Here's how the part is built. I have some questions about the finished solid (model axes, mm). Face numbers are marked on the shaded views. A direction names the side the tool comes from. Round coordinates to 2 decimals unless told otherwise and drop trailing zeros. Order: outer loops, then holes, each group sorted by start corner. A loop starts at its lowest first (then second) coordinate and runs counter-clockwise, first axis right, second up.
```python
from build123d import *

# Parameters (mm, degrees)
ESQUISSE1_R             = 40
ESQUISSE1_R_2           = 10
BOSS_EXTRU_1_DEPTH      = 12.5
ESQUISSE2_R             = 22.5
ENL_V_MAT_EXTRU_1_DEPTH = 5
CHANFREIN1_SIZE         = 5
ESQUISSE4_R             = 3
ENL_V_MAT_EXTRU_2_DEPTH = 61
BOSS_EXTRU_2_DEPTH      = 2
BOSS_EXTRU_2_DEPTH_BACK = 17
ESQUISSE5_R             = 11
ESQUISSE5_R_2           = 10
CHANFREIN2_SIZE         = 0.5
ESCALA1_SCALE           = 0.7916


with BuildPart() as part:
    # Esquisse1 → Boss.-Extru.1 (new, symmetric)
    with BuildSketch(Plane.XY):
        Circle(ESQUISSE1_R)
        Circle(ESQUISSE1_R_2, mode=Mode.SUBTRACT)
    extrude(amount=BOSS_EXTRU_1_DEPTH, both=True)

    # Esquisse2 → Enlèv. mat.-Extru.1 (cut)
    with BuildSketch(Plane.XY.offset(12.5)):
        Circle(ESQUISSE2_R)
    enl_v_mat_extru_1 = extrude(amount=-ENL_V_MAT_EXTRU_1_DEPTH, mode=Mode.SUBTRACT)

    # Symétrie1: Enlèv. mat.-Extru.1 across plane
    add(enl_v_mat_extru_1.mirror(Plane.XY), mode=Mode.SUBTRACT)

    # Esquisse3 → Enlèvement de matière-Révolution1 (revolve, cut)
    with BuildSketch(Plane(origin=(0, 0, 0), x_dir=(1, 0, 0), z_dir=(0, 1, 0))):
        Polygon((40, 9.5), (34, 6.035898385), (34, -6.035898385), (40, -9.5), align=None)
    revolve(axis=Axis((0, 0, 0), (0, 0, -1)), mode=Mode.SUBTRACT)

    # Chanfrein1
    chanfrein1_edges = [part.edges().sort_by_distance(p)[0] for p in [
        (-22.5, 0, 12.5),
        (-22.5, 0, -12.5),
    ]]
    chamfer(chanfrein1_edges, length=CHANFREIN1_SIZE - 0.0001)  # a hair under: the kernel refuses the full size

    # Esquisse4 → Enlèv. mat.-Extru.2 (cut, through all)
    with BuildSketch(Plane(origin=(0, 0, -7.5), x_dir=(-1, 0, 0), z_dir=(0, 0, -1))):
        with Locations((0, 17)):
            Circle(ESQUISSE4_R)
        with Locations((14.722431864, -8.5)):
            Circle(ESQUISSE4_R)
        with Locations((-14.722431864, -8.5)):
            Circle(ESQUISSE4_R)
    extrude(amount=-ENL_V_MAT_EXTRU_2_DEPTH, mode=Mode.SUBTRACT)

    # Esquisse5 → Boss.-Extru.2 (add, two sides: drawn at the far end of the back side and taken through both)
    with BuildSketch(Plane(origin=(0, 0, -7.5), x_dir=(-1, 0, 0), z_dir=(0, 0, -1)).offset(-BOSS_EXTRU_2_DEPTH_BACK)):
        Circle(ESQUISSE5_R)
        Circle(ESQUISSE5_R_2, mode=Mode.SUBTRACT)
    extrude(amount=BOSS_EXTRU_2_DEPTH + BOSS_EXTRU_2_DEPTH_BACK)

    # Chanfrein2
    chanfrein2_edges = [part.edges().sort_by_distance(p)[0] for p in [
        (10, 0, 9.5),
        (10, 0, -9.5),
    ]]
    chamfer(chanfrein2_edges, length=CHANFREIN2_SIZE)


with BuildPart() as part_1:
    # Escala1: scaled about (0, 0, 0)
    add(part.part.scale(ESCALA1_SCALE))


solid = part_1.part
```
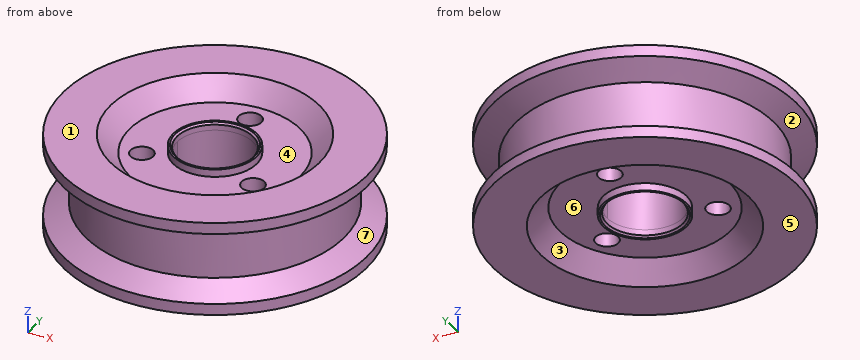
1) I need wall thicknesses on line 1 (X direction, y = 0, z = -6.45); line 2 (X direction, y = 0, z = -6.65); line 3 (Z direction, x = -11, y = 1). Which ranges of each line are inside material? Lowest first, please.
2) For the marked faces 4, 5, 6 and 7, which set-ups out of +Z, -Z, +X, -X, +Y, -Y let a thin tool reach every point of the face, with its end or its side?
3) I'm going to push flat-ended pins straight in: pin 1 (19 mm diameter, centred on x = 3, y = -0.5, fed in from -Z); pin 2 (6 mm diameter, centred on x = 25, z = -7, fed in from -Y); pin 3 (14 mm diameter, centred on x = 2.5, y = -1.5, fed in from +Z). Where does each tip first touch, or does it pass through?
4) If we section it at A-A (x = 0): Give the number of separate pieces and of enclosed holes in the cut face, plus the area to 3 significant figures.
5) We'd pull the mould along X, two halves only. Please class the marked faces 1, 2 and 3: +X half, -X half, draft (parallel to the pull), parting line (faces both ways), or undercut.
6) If we section it at B-B (z = 4): Write out the boundary of the cut face in (x, y), plus the area to 3 significant figures.
Solutions:
1. line 1: x = -29.81 to -18.32, -8.71 to -7.92, 7.92 to 8.71, 18.32 to 29.81
1. line 2: x = -30.16 to -18.52, -8.71 to -7.92, 7.92 to 8.71, 18.52 to 30.16
1. line 3: z = -5.94 to 5.94
2. face 4: +Z
2. face 5: -Z, +X, -X, +Y, -Y
2. face 6: -Z
2. face 7: none
3. pin 1: stops at z = -7.52
3. pin 2: stops at y = -22.73
3. pin 3: stops at z = 7.52
4. separate pieces: 3
4. enclosed holes: 0
4. area: 583 mm2
5. face 1: draft
5. face 2: parting line
5. face 3: undercut
6. outline: circle Ø53.83 at (0, 0); hole circle Ø4.75 at (-11.65, -6.73); hole circle Ø15.83 at (0, 0); hole circle Ø4.75 at (0, 13.46); hole circle Ø4.75 at (11.65, -6.73)
6. area: 2,030 mm2
